Verification items for this drawing (mm, ordinates from the low corner). A direction names the side the tool comes from. Give positions to 0.01 mm unless a question says otherwise; leave off trailing zeros. Loops run counter-clockwise (first coordinate to the right, second up) from the corner with the lowest first, then second, coordinate; pieces in that order, holes last. Notation, with made-up numbers: (78.5, 68.5) -> (102.5, 68.5) arc R33 cw to (102.5, 97.5) -> close; hole circle Ø5 at (-32, -17). An arc over 180 degrees is marked (long way). Write each question's results on one line, items separated by ' | '. Start each with the question number.
Item 1: Cross-section at A-A on z = 12. Enter the section's corners in (x, y).
Item 2: Cross-section at D-D on z = 23.5. Enter the section's corners in (x, y), then the cut area to 3 significant figures.
Item 3: Mould release check, pull along X, two halves, no side actions. Record for the marked faces 1, 2, 3 and 4: pulls with the +X half, pulls with the -X half, needs draft (parallel to the pull), parting line crosses it, or undercut.
Item 4: Scan lines: line 1 along Y through (x, z) = (22, 14); line 2 along Z through (x, y) = (10, 122.5). Record each from-to range of solid material in increasing order.
Item 5: Gauge pin test, flat ends, axial feed: pin 1 Ø6 at (x, z) = (10, 25) entering from +Y; pin 2 Ø3 at (x, y) = (23, 109.5) entering from +Z; pin 3 Ø6 at (x, z) = (12.5, 14) entering from -Y; pin 4 Ø3 at (y, z) = (61, 7.5) entering from -X. Record the tip position at first contact, or that the pin passes through.
Item 6: Access from +Z, -Z, +X, -X, +Y, -Y to the whole of each face (thin tool, end or side, straight path). Record for the marked faces 5, 6 and 7.
Item 7: Cross-section at B-B on x = 10. Enter the section's corners in (y, z).
Item 8: Cross-section at C-C on x = 22. Enter the section's corners in (y, z).
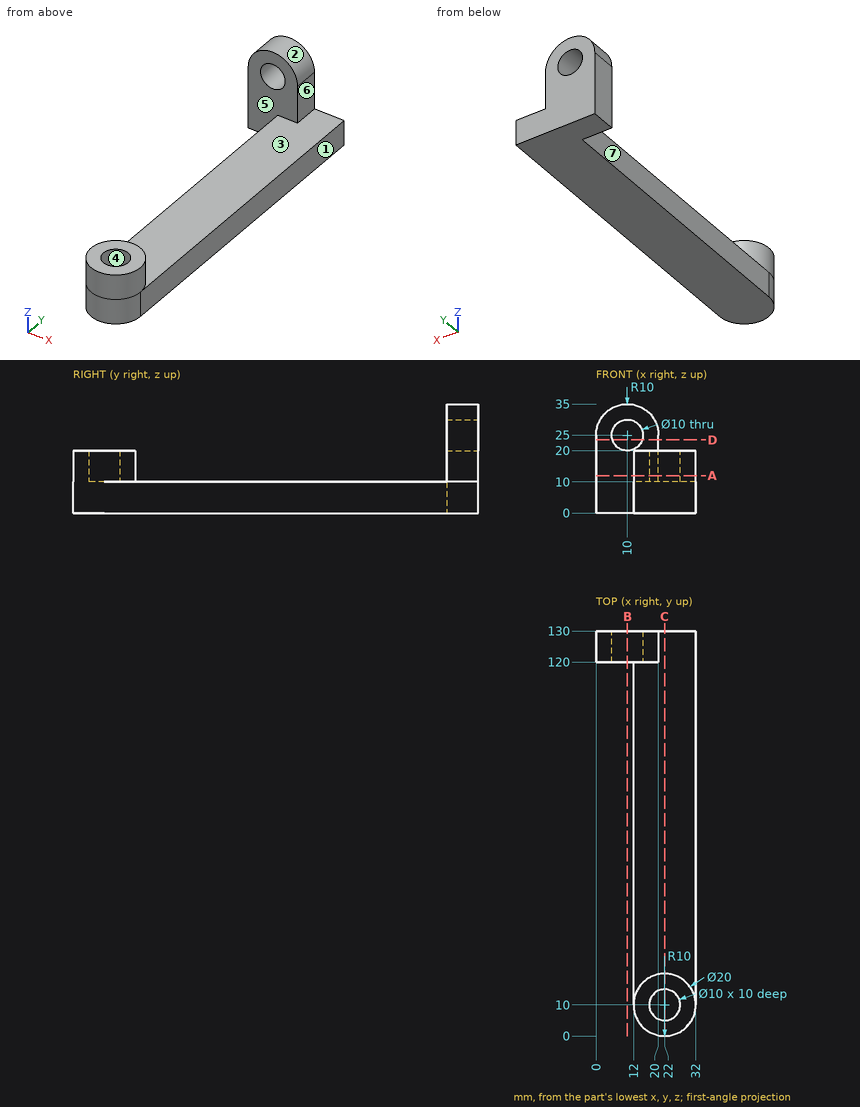
Answer sheet:
1) outline: (0, 120) -> (20, 120) -> (20, 130) -> (0, 130) -> close; circle Ø20 at (22, 10); hole circle Ø10 at (22, 10)
2) outline: (0, 120) -> (5.23, 120) -> (5.23, 130) -> (0, 130) -> close; (14.77, 120) -> (20, 120) -> (20, 130) -> (14.77, 130) -> close | area: 105 mm²
3) face 1: pulls with the +X half | face 2: parting line crosses it | face 3: needs draft | face 4: undercut
4) line 1: y = 0 to 5, 15 to 20 | line 2: z = 0 to 20, 30 to 35
5) pin 1: passes through | pin 2: stops at z = 10 | pin 3: stops at y = 2.4 | pin 4: stops at x = 12
6) face 5: +Z, -X | face 6: +Z, +X, +Y | face 7: +Z, -Z, -X, -Y
7) outline: (120, 0) -> (130, 0) -> (130, 20) -> (120, 20) -> close; (120, 30) -> (130, 30) -> (130, 35) -> (120, 35) -> close
8) outline: (0, 0) -> (130, 0) -> (130, 10) -> (20, 10) -> (20, 20) -> (15, 20) -> (15, 10) -> (5, 10) -> (5, 20) -> (0, 20) -> close
